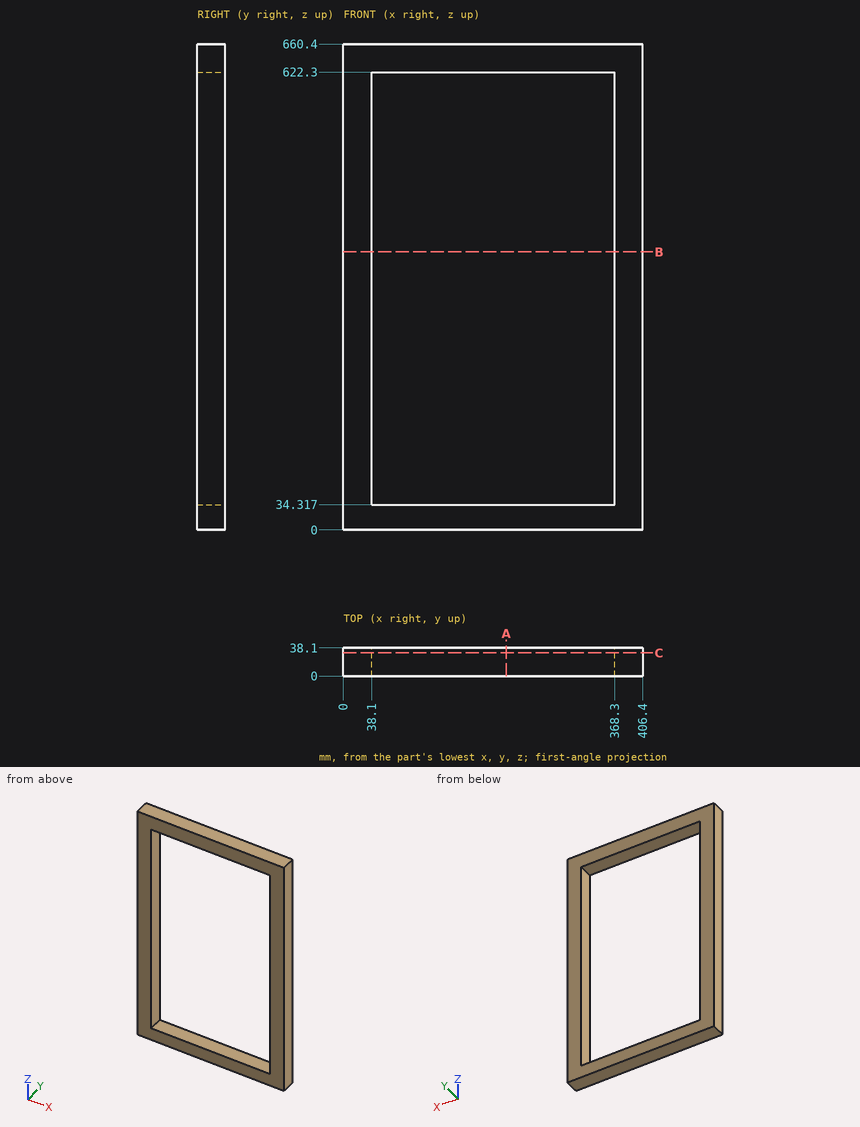
Answer from the drawing. Dimensions are ordinates in mm from the lowest x, y and z of the part. Round coordinates to 2 decimals unless told otherwise and drop trailing zeros. Order: outer loops, then holes, each group sorted by start corner. A loop starts at its lowest first (then second) coordinate and runs counter-clockwise, first axis right, second up. Notation, with made-up numbers: (71.25, 66.5) - (107.25, 66.5) arc R9 ccw to (107.25, 81.5) - close; hole circle Ø7 at (8, -21). An arc over 180 degrees is marked (long way). Put each result on its own line as item: value. Start each with the question number.
(1) Straight lines are drawn through the part: probe 1 along Z at (x, y) = (109, 20); probe 2 along X at (y, z) = (21.5, 242). For each, find the intervals that lie inside material, in ascending order. Write a range as from..to.
(2) Find section A-A (x = 221.5). Give the vertices of the cut face in (y, z).
(3) Find section B-B (z = 378). Give the vertices of the cut face in (x, y).
(4) Find section C-C (y = 31.5). Give the vertices of the cut face in (x, z), plus the area to 3 significant figures.
Reply:
1. probe 1: 0..34.32, 622.3..660.4
1. probe 2: 0..38.1, 368.3..406.4
2. outline: (0, 0) - (38.1, 0) - (38.1, 34.32) - (0, 34.32) - close; (0, 622.3) - (38.1, 622.3) - (38.1, 660.4) - (0, 660.4) - close
3. outline: (0, 0) - (38.1, 0) - (38.1, 38.1) - (0, 38.1) - close; (368.3, 0) - (406.4, 0) - (406.4, 38.1) - (368.3, 38.1) - close
4. outline: (0, 0) - (406.4, 0) - (406.4, 660.4) - (0, 660.4) - close; hole (38.1, 34.32) - (368.3, 34.32) - (368.3, 622.3) - (38.1, 622.3) - close
4. area: 74,200 mm^2
